For this review, use the dimensioned drawing (mm, ordinates from the lowest corner) and the shaded views. Give positions to 0.01 mm unless a question says otherwise; leave off trailing zeros.
1) Draft analysis for pull direction Y (two halves, no side actions). For the marked faces 1, 2, 3 and 4, state which applies: pulls with the +Y half, pulls with the -Y half, needs draft (parallel to the pull), parting line crosses it, or undercut.
2) For P1, Ø2, axis at x = 7, y = 11, coming from the -Z side; P2, Ø2.5, axis at x = 3.5, y = 26.5, coming from the -Z side, all flat-tipped, find the tip position at first contact; note any pin that passes through.
3) Wall thickness on line 1 along Y through (x, z) = (4, 5) (1 decimal); line 2 along Z through (x, y) = (6.5, 3) (1 decimal); line 3 along Z through (x, y) = (6, 3.5) (1 decimal): over which ranges is each line inside the solid? List them lowest first.
4) We need section A-A on z = 5.75. Give the number of separate pieces and of enclosed holes in the cut face, and give its area (3 significant figures).
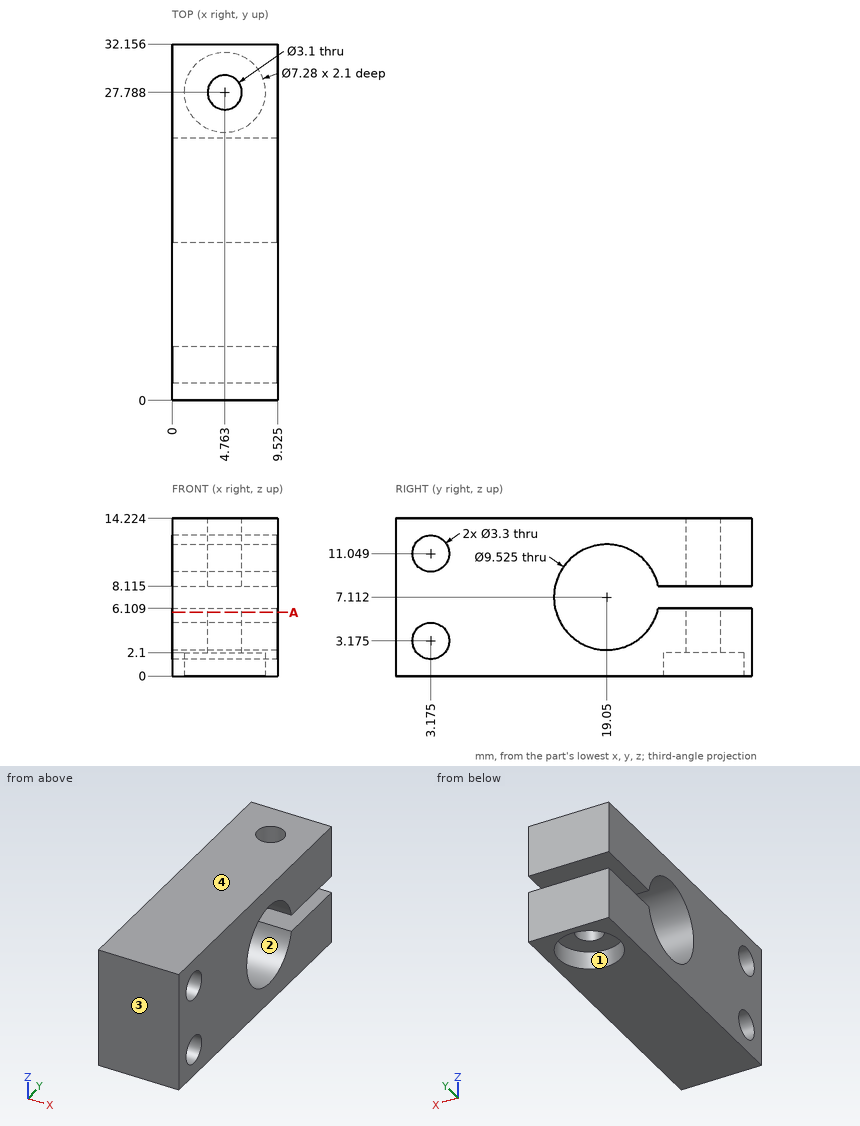
Results list:
1. face 1: undercut
1. face 2: undercut
1. face 3: pulls with the -Y half
1. face 4: needs draft
2. P1: stops at z = 0
2. P2: stops at z = 2.1
3. line 1: y = 0 to 14.8, 23.3 to 26.4, 29.1 to 32.2
3. line 2: z = 0 to 1.5, 4.8 to 9.4, 12.7 to 14.2
3. line 3: z = 0 to 1.6, 4.8 to 9.4, 12.7 to 14.2
4. separate pieces: 2
4. enclosed holes: 1
4. area: 212 mm2
